Can you work these out from the model? Positions are in its coordinate system, mm. Face numbers are marked on the shaded views. A direction names the side the tool comes from. Coordinates: 2 decimals unless noted, no trailing zeros. Loops run counter-clockwise (first coordinate to the right, second up) from the corner with the lowest first, then second, coordinate; pieces in that order, holes last.
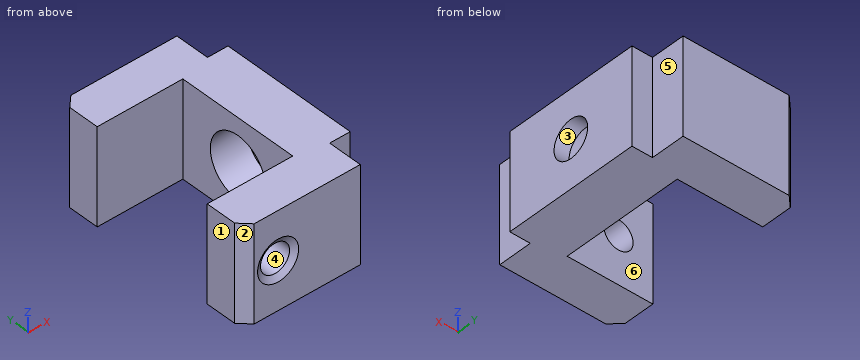
```python
from build123d import *

# Parameters (mm, degrees)
BOSS_EXTRU_1_DEPTH                                 = 28
CHANFREIN1_SIZE                                    = 3
CHAMBRAGE_POUR_VIS_T_TE_HEXAGONALE_M10_D           = 11
CHAMBRAGE_POUR_VIS_T_TE_HEXAGONALE_M10_CBORE_D     = 18
CHAMBRAGE_POUR_VIS_T_TE_HEXAGONALE_M10_CBORE_DEPTH = 10.6


with BuildPart() as part:
    # Esquisse1 → Boss.-Extru.1 (new body)
    with BuildSketch(Plane.XY):
        Polygon((0, 0), (0, 10), (6, 10), (6, 50), (0, 50), (0, 60), (-34, 60), (-34, 48), (-9, 48), (-9, 12), (-34, 12), (-34, 0), align=None)
    extrude(amount=BOSS_EXTRU_1_DEPTH)

    # Chanfrein1
    chanfrein1_edges = [part.edges().sort_by_distance(p)[0] for p in [
        (-34, 0, 14),
        (-34, 60, 14),
    ]]
    chamfer(chanfrein1_edges, length=CHANFREIN1_SIZE)

    # Esquisse3 → Trou taraudé M101 (revolve, cut)
    with BuildSketch(Plane(origin=(-24, 12, 14), x_dir=(0, 0, 1), z_dir=(1, 0, 0))):
        Polygon((0, 0), (0, 12), (6, 12), (4.25, 10.989637029), (4.25, 0), align=None)
    revolve(axis=Axis((-24, 18.35, 14), (0, -1, 0)), mode=Mode.SUBTRACT)

    # Chambrage pour vis à tête hexagonale M101 (through all)
    with Locations(Plane.ZY.offset(9)):
        with Locations((14, 30)):
            CounterBoreHole(CHAMBRAGE_POUR_VIS_T_TE_HEXAGONALE_M10_D / 2, CHAMBRAGE_POUR_VIS_T_TE_HEXAGONALE_M10_CBORE_D / 2, CHAMBRAGE_POUR_VIS_T_TE_HEXAGONALE_M10_CBORE_DEPTH)


solid = part.part
```
(1) Which directions (+Z, -Z, +X, -X, +Y, -Y) give clear straight access to the entire face, cutting with the end or side of a thin tool? Please do the marked faces 4, 5 and 6.
Check values:
face 4: -Y
face 5: +Z, -Z, +X, +Y
face 6: +Z, -Z, -X
(2) If we mould it in two halves opening along Y, with no side actions, what happens to the marked faces 1, 2 and 3? For each: released by +Y, released by -Y, zero draft, split by the parting line, or undercut.
Check values:
face 1: zero draft
face 2: released by -Y
face 3: undercut
(3) I'm going to push flat-ended pins straight in: pin 1 (6.5 mm diameter, centred on y = 30, z = 14, fed in from +X); pin 2 (12 mm diameter, centred on x = -5.5, y = 46, fed in from -Z); pin 3 (8.5 mm diameter, centred on y = 23.5, z = 12.5, fed in from -X); pin 4 (11 mm diameter, centred on x = -24, z = 14, fed in from -Y). Where does each tip first touch, or does it pass through?
Check values:
pin 1: passes through
pin 2: stops at z = 0
pin 3: stops at x = -9
pin 4: stops at y = 0.29
(4) I want a section at A-A on y = 30. Write out the boundary of the cut face in (x, z), then the cut area to 3 significant figures.
Check values:
outline: (-9, 0) - (6, 0) - (6, 8.5) - (1.6, 8.5) - (1.6, 5) - (-9, 5) - close; (-9, 23) - (1.6, 23) - (1.6, 19.5) - (6, 19.5) - (6, 28) - (-9, 28) - close
area: 181 mm2
(5) If I drill on probe 1 along Y at (x, z) = (-24, 4); probe 2 along Y at (x, z) = (4.4, 14); probe 3 along X at (y, z) = (4.25, 14), over which ranges is the centre line in solid material (lowest first)?
Check values:
probe 1: y = 0 to 12, 48 to 60
probe 2: y = 10 to 24.5, 35.5 to 50
probe 3: x = -34 to -28.25, -19.75 to 0
(6) I want a section at D-D on x = -10. Write out the boundary of the cut face in (y, z), then the cut area to 3 significant figures.
Check values:
outline: (0, 0) - (12, 0) - (12, 28) - (0, 28) - close; (48, 0) - (60, 0) - (60, 28) - (48, 28) - close
area: 672 mm2
(7) I want a section at B-B on z = 14. Write out the boundary of the cut face in (x, y), then the cut area to 3 significant figures.
Check values:
outline: (-34, 3) - (-31, 0) - (-30, 0) - (-28.25, 1.01) - (-28.25, 12) - (-34, 12) - close; (-34, 48) - (-9, 48) - (-9, 39) - (1.6, 39) - (1.6, 35.5) - (6, 35.5) - (6, 50) - (0, 50) - (0, 60) - (-31, 60) - (-34, 57) - close; (-19.75, 1.01) - (-18, 0) - (0, 0) - (0, 10) - (6, 10) - (6, 24.5) - (1.6, 24.5) - (1.6, 21) - (-9, 21) - (-9, 12) - (-19.75, 12) - close
area: 1,030 mm2
(8) I want a section at C-C on x = -24. Write out the boundary of the cut face in (y, z).
Check values:
outline: (0, 0) - (12, 0) - (12, 9.75) - (1.01, 9.75) - (0, 8) - close; (0, 20) - (1.01, 18.25) - (12, 18.25) - (12, 28) - (0, 28) - close; (48, 0) - (60, 0) - (60, 28) - (48, 28) - close
